Print and shaded views of the part. All mm, measured from the part's lowest x, y and z. Round coordinates to 2 decimals unless told otherwise and drop trailing zeros. Order: outer loops, then holes, each group sorted by start corner. A loop starts at its lowest first (then second) coordinate and runs counter-clockwise, first axis right, second up. Notation, with made-up numbers: (79.5, 69) - (135.5, 69) arc R36 ccw to (135.5, 107) - close; hole circle Ø2 at (-36, 12.25). An arc over 180 degrees is marked (long way). Return JSON: item names as keys, results as strings. Group by question number.
Item 1: Probe probe 1 along X at (y, z) = (8.5, 26) (1 decimal); probe 2 along Y at (x, z) = (5, 23.5) (1 decimal). List the from-to ranges inside material, lowest first.
Item 2: Drop flat-ended pins along their axis: pin 1 (1.5 mm diameter, centred on x = 5, y = 8.5, fed in from -Z); pin 2 (4 mm diameter, centred on x = 27, y = 6.5, fed in from +Z); pin 3 (4 mm diameter, centred on y = 3, z = 20, fed in from +X). Give the stop position or say it passes through.
Item 3: Saw through at D-D on y = 2.75. List the corners of the cut face in (x, z) (1 decimal).
Item 4: Saw through at C-C on x = 43.5. List the corners of the cut face in (y, z) (1 decimal).
Item 5: Two-plate mould, pull along X, no slides. Class the marked faces 1, 2 and 3: released by +X, released by -X, zero draft, split by the parting line, or undercut.
Item 6: Saw through at A-A on z = 37. List the corners of the cut face in (x, y) (1 decimal).
Item 7: Saw through at B-B on x = 9.5. List the corners of the cut face in (y, z) (1 decimal), and give its area (3 significant figures).
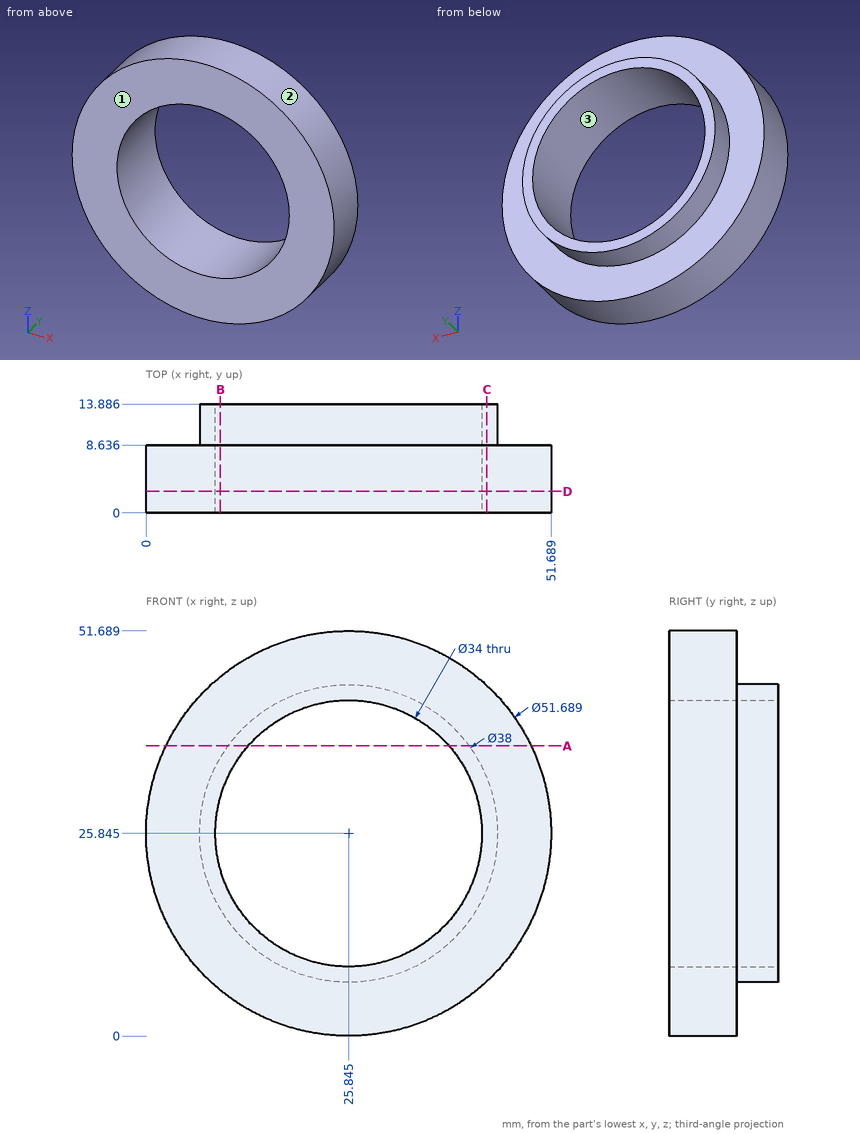
Filled in:
{
 "1": {"probe 1": "x = 0 to 8.8, 42.8 to 51.7", "probe 2": "y = 0 to 8.6"},
 "2": {"pin 1": "stops at z = 9.59", "pin 2": "stops at z = 51.69", "pin 3": "stops at x = 51.4"},
 "3": {"outline": "circle Ø51.7 at (25.8, 25.8); hole circle Ø34 at (25.8, 25.8)"},
 "4": {"outline": "(0, 7) - (8.6, 7) - (8.6, 18.8) - (13.9, 18.8) - (13.9, 32.9) - (8.6, 32.9) - (8.6, 44.7) - (0, 44.7) - close"},
 "5": {"face 1": "zero draft", "face 2": "split by the parting line", "face 3": "undercut"},
 "6": {"outline": "(2.5, 0) - (13, 0) - (13, 13.9) - (10.5, 13.9) - (10.5, 8.6) - (2.5, 8.6) - close; (38.7, 0) - (49.2, 0) - (49.2, 8.6) - (41.2, 8.6) - (41.2, 13.9) - (38.7, 13.9) - close"},
 "7": {"outline": "(0, 5.8) - (8.6, 5.8) - (8.6, 16.2) - (13.9, 16.2) - (13.9, 21.2) - (0, 21.2) - close; (0, 30.5) - (13.9, 30.5) - (13.9, 35.5) - (8.6, 35.5) - (8.6, 45.9) - (0, 45.9) - close", "area": "318 mm^2"}
}
